Autodesk Inventor part; units mm, degrees
ref_plane "YZ Plane" through (0, 0, 0) normal (1, 0, 0) x (0, 1, 0)
ref_plane "XZ Plane" through (0, 0, 0) normal (0, 1, 0) x (-1, 0, 0)
ref_plane "XY Plane" through (0, 0, 0) normal (0, 0, 1) x (1, 0, 0)
sketch "Sketch1" plane through (0, 0, 0) normal (0, 1, 0) x (-1, 0, 0)
  line L0 (-14.478, 12.7) -> (14.478, 12.7)
  line L1 (14.478, 12.7) -> (14.478, -12.7)
  line L2 (14.478, -12.7) -> (-14.478, -12.7)
  line L3 (-14.478, -12.7) -> (-14.478, 12.7)
  line L4 (-14.478, 12.7) -> (14.478, -12.7) construction
  line L5 (14.478, 12.7) -> (-14.478, -12.7) construction
  point P0 (0, 0)
  dimension "d0" = 28.956
  dimension "d1" = 25.4
extrude "Extrusion1" add sketch "Sketch1" along normal blind 12.7
sketch "Sketch2" plane through (0, 12.7, 0) normal (0, 1, 0) x (1, 0, 0)
  point P0 (0, 0)
  point P1 (0, -9.779)
  point P2 (0, 9.779)
  dimension "d4" = 9.779
  dimension "d5" = 19.558
hole "Hole1" at (0, 12.7, 9.779) at (0, 12.7, -9.779) direction (0, -1, 0) diameter 3.81 end through all
sketch "Sketch3" plane through (14.478, 0, 12.7) normal (1, 0, 0) x (0, 0, -1)
  circle A0 centre (12.7, 6.35) radius 1.5
  line L0 (25.4, 0) -> (0, 0)
  line L1 (0, 12.7) -> (25.4, 12.7)
  point P0 (12.7, 0)
  point P1 (12.7, 0)
  point P2 (11.582, 7.35)
  point P3 (13.818, 7.35)
  dimension "d13" = 3
  dimension "d14" = 6.35
  dimension "d15" = 12.7
extrude "Extrusion3" cut sketch "Sketch3" against normal through all
sketch "Sketch5" plane through (-14.478, 0, -12.7) normal (-1, 0, 0) x (0, 0, 1)
  line L0 (6.604, 1.27) -> (18.796, 1.27)
  line L1 (18.796, 1.27) -> (18.796, 11.43)
  line L2 (18.796, 11.43) -> (6.604, 11.43)
  line L3 (6.604, 11.43) -> (6.604, 1.27)
  line L4 (6.604, 1.27) -> (18.796, 11.43) construction
  line L5 (18.796, 1.27) -> (6.604, 11.43) construction
  line L6 (0, 12.7) -> (25.4, 12.7)
  line L7 (25.4, 0) -> (0, 0)
  point P0 (12.7, 0)
  point P1 (12.7, 6.35)
  dimension "d23" = 12.192
  dimension "d24" = 10.16
  dimension "d25" = 1.27
  dimension "d26" = 1.27
extrude "Extrusion5" cut sketch "Sketch5" against normal blind 27.94
equation "\"d26\" = d25"
properties part number "MotorEnclosure" material "ABS Plastic"
For this review, take the finished solid that the model builds, in its own axes (mm). A direction names the side the tool comes from. Round coordinates to 2 decimals unless told otherwise and drop trailing zeros. Write each loop counter-clockwise with the first axis right and the second up, starting at its lowest first coordinate (ties: lowest second). Pieces come first, ordered by that corner, then holes. Notation, with made-up numbers: (15, 76.5) -> (31, 76.5) arc R33 ccw to (31, 104.5) -> close; hole circle Ø8 at (56.5, -29.75). An arc over 180 degrees is marked (long way). One line per question, with ' | ' between items. Start each with the question number.
1) For pin 1 Ø1.5 at (y, z) = (7, -2.5) entering from -X, flat-tipped, find the tip position at first contact; note if it passes through.
2) Add section D-D (x = -12). Write out the cut boundary in (y, z), and give its area (3 significant figures).
3) Wall thickness on line 1 along Z through (x, y) = (12.75, 5.5); line 2 along Z through (x, y) = (0, 5.5); line 3 along Y through (x, z) = (-7.75, -3.5): over which ranges is each line inside the solid? List them lowest first.
4) Machinability: for faces 1 (the flat face through (-1, 6, -6.096)), 2 (the cylindrical face through (0.73, 6.26, -8.02)), which of the approach directions +Z, -Z, +X, -X, +Y, -Y give a long, thin tool a straight path to every point of the face, cutting with its end or side? Answer none if there is none.
5) Add section C-C (x = 0). Write out the cut boundary in (y, z), and give its area (3 significant figures).
6) Mouldability with a two-part tool opening along Y and no side actions: class faces 3 (the flat face through (0, 0, 0)), 4 (the flat face through (14.478, 3, 0)), 5 (the cylindrical face through (13.977, 7.615, -0.806)), 6 (the flat face through (-1, 1.27, 0)) as +Y half, -Y half, draft (parallel to the pull), parting line (faces both ways), or undercut.
7) Add section A-A (z = 0). Write out the cut boundary in (x, y).
8) Add section B-B (y = 6.35). Write out the cut boundary in (x, z) (3 decimals), and give its area (3 significant figures).
Reported:
1) pin 1: stops at x = 13.46
2) outline: (0, -12.7) -> (12.7, -12.7) -> (12.7, 12.7) -> (0, 12.7) -> close; hole (1.27, -6.1) -> (11.43, -6.1) -> (11.43, 6.1) -> (1.27, 6.1) -> close | area: 199 mm²
3) line 1: z = -12.7 to -6.1, 6.1 to 12.7 | line 2: z = -12.7 to -11.68, -7.87 to -6.1, 6.1 to 7.87, 11.68 to 12.7 | line 3: y = 0 to 1.27, 11.43 to 12.7
4) face 1: -X | face 2: +Y, -Y
5) outline: (0, -12.7) -> (12.7, -12.7) -> (12.7, -11.68) -> (0, -11.68) -> close; (0, -7.87) -> (12.7, -7.87) -> (12.7, 7.87) -> (0, 7.87) -> close; (0, 11.68) -> (12.7, 11.68) -> (12.7, 12.7) -> (0, 12.7) -> close; hole (1.27, -6.1) -> (11.43, -6.1) -> (11.43, 6.1) -> (1.27, 6.1) -> close | area: 102 mm²
6) face 3: -Y half | face 4: draft | face 5: undercut | face 6: undercut
7) outline: (-14.48, 0) -> (14.48, 0) -> (14.48, 4.85) -> (13.46, 4.85) -> (13.46, 1.27) -> (-14.48, 1.27) -> close; (-14.48, 11.43) -> (13.46, 11.43) -> (13.46, 7.85) -> (14.48, 7.85) -> (14.48, 12.7) -> (-14.48, 12.7) -> close
8) outline: (-14.478, -12.7) -> (14.478, -12.7) -> (14.478, -1.5) -> (13.462, -1.5) -> (13.462, -6.096) -> (-14.478, -6.096) -> close; (-14.478, 6.096) -> (13.462, 6.096) -> (13.462, 1.5) -> (14.478, 1.5) -> (14.478, 12.7) -> (-14.478, 12.7) -> close; hole circle Ø3.81 at (0, -9.779); hole circle Ø3.81 at (0, 9.779) | area: 369 mm²
